Could you check a few things on this model? Use its own coordinates, in mm. Face numbers are marked on the shaded views. Coordinates: 2 decimals unless noted, no trailing zeros. Loops run counter-clockwise (first coordinate to the right, second up) from the corner with the lowest first, then second, coordinate; pieces in that order, holes last.
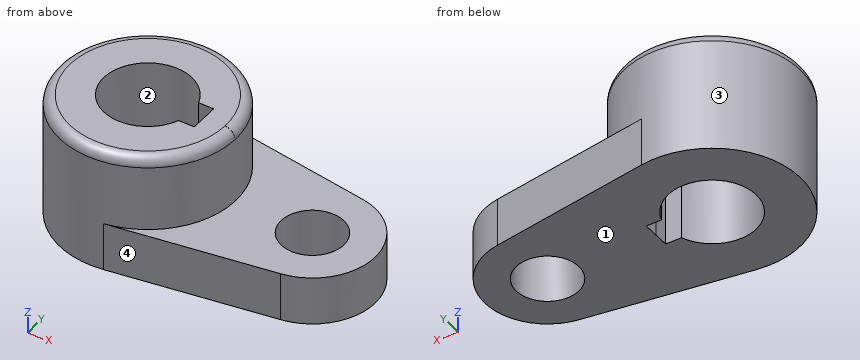
from build123d import *

# Parameters (mm, degrees)
F1_DEPTH = 15.7734
F2_DEPTH = 40.2336
F3_R     = 3.302


# Not quite as in the source:
# - a feature names something its author has since deleted; it is built from what else it names


with BuildPart() as f1:
    # F0 (on Top) → F1 (new body)
    with BuildSketch(Plane.XY):
        with BuildLine():
            ThreePointArc((28.5749057346, -0.0733979643), (28.5749764336, -0.0366990124), (28.575, 0))
            ThreePointArc((28.575, 0), (21.7196871584, 18.5684090525), (4.4430094671, 28.2274740612))
            ThreePointArc((4.4430094671, 28.2274740612), (-28.5749057039, 0.0734099128), (4.2979170796, -28.2499298013))
            ThreePointArc((4.2979170796, -28.2499298013), (21.6479758068, -18.6519641987), (28.5749057346, -0.0733979643))
        make_face()
        with BuildLine():
            Line((18.4686649637, 4.6872641706), (18.4984100104, -0.0475153147))
            Line((18.4984100104, -0.0475153147), (18.5293, -4.9645453691))
            Line((18.5293, -4.9645453691), (13.3852167998, -4.9968617623))
            ThreePointArc((13.3852167998, -4.9968617623), (-14.2863531341, 0.1810259026), (13.5075318215, 4.6560971147))
            Line((13.5075318215, 4.6560971147), (18.4686649637, 4.6872641706))
        make_face(mode=Mode.SUBTRACT)
        with BuildLine():
            ThreePointArc((4.4430094671, 28.2274740612), (21.7196871584, 18.5684090525), (28.575, 0))
            ThreePointArc((28.575, 0), (28.5749764336, -0.0366990124), (28.5749057346, -0.0733979643))
            ThreePointArc((28.5749057346, -0.0733979643), (21.6479758068, -18.6519641987), (4.2979170796, -28.2499298013))
            Line((4.2979170796, -28.2499298013), (56.9175468923, -20.2444300608))
            ThreePointArc((56.9175468923, -20.2444300608), (74.2947643422, -0.1870234197), (57.0132588055, 19.9529074106))
            Line((57.0132588055, 19.9529074106), (4.4430094671, 28.2274740612))
        make_face()
        with BuildLine():
            ThreePointArc((64.1348219431, -0.1386405993), (53.9617734053, -10.2986322201), (43.8148554597, -0.1125435453))
            ThreePointArc((43.8148554597, -0.1125435453), (53.9878704808, 10.0213510216), (64.1348219431, -0.1386405993))
        make_face(mode=Mode.SUBTRACT)
    extrude(amount=F1_DEPTH)

    # F0 (on Top) → F2 (join)
    with BuildSketch(Plane.XY):
        with BuildLine():
            ThreePointArc((28.5749057346, -0.0733979643), (28.5749764336, -0.0366990124), (28.575, 0))
            ThreePointArc((28.575, 0), (21.7196871584, 18.5684090525), (4.4430094671, 28.2274740612))
            ThreePointArc((4.4430094671, 28.2274740612), (-28.5749057039, 0.0734099128), (4.2979170796, -28.2499298013))
            ThreePointArc((4.2979170796, -28.2499298013), (21.6479758068, -18.6519641987), (28.5749057346, -0.0733979643))
        make_face()
        with BuildLine():
            Line((18.4686649637, 4.6872641706), (18.4984100104, -0.0475153147))
            Line((18.4984100104, -0.0475153147), (18.5293, -4.9645453691))
            Line((18.5293, -4.9645453691), (13.3852167998, -4.9968617623))
            ThreePointArc((13.3852167998, -4.9968617623), (-14.2863531341, 0.1810259026), (13.5075318215, 4.6560971147))
            Line((13.5075318215, 4.6560971147), (18.4686649637, 4.6872641706))
        make_face(mode=Mode.SUBTRACT)
    extrude(amount=F2_DEPTH)

    # F3
    f3_edges = [f1.edges().sort_by_distance(p)[0] for p in [
        (-4.297917, 28.24993, 40.2336),
    ]]
    fillet(f3_edges, radius=F3_R)


solid = f1.part
1) Imagine slicing it at D-D on x = 34. List the corners of the cut face in (y, z) for me, plus the area to 3 significant figures.
2) Imagine slicing it at B-B on z = 5.5. State how many separate pieces and enclosed holes the cut face has, plus the area to 3 significant figures.
3) If I drill on L1, parallel to X at y = 0, z = 13 (1 decimal); L2, parallel to Y at x = 0, z = 9 (1 decimal); L3, parallel to X at y = 8, z = 25, over which ranges is the centre line in solid material (lowest first)?
4) We'd pull the mould along Y, two halves only. Please class the marked faces 1, 2, 3 and 4: released by +Y, released by -Y, zero draft, split by the parting line, or undercut.
5) Will these pins go through, and if not, where does the flat tip stop? pin 1 (5 mm diameter, centred on y = 16, z = 24, fed in from -X); pin 2 (5 mm diameter, centred on y = 20.5, z = 14.5, fed in from -X); pin 3 (5 mm diameter, centred on x = 61.5, z = 12, fed in from +Y).
Solved:
1. outline: (-23.73, 0) - (23.58, 0) - (23.58, 15.77) - (-23.73, 15.77) - close
1. area: 746 mm2
2. separate pieces: 1
2. enclosed holes: 2
2. area: 3,590 mm2
3. L1: x = -28.6 to -14.3, 18.5 to 43.8, 64.1 to 74.3
3. L2: y = -28.6 to -14.3, 14.3 to 28.6
3. L3: x = -27.43 to -11.84, 11.84 to 27.43
4. face 1: zero draft
4. face 2: undercut
4. face 3: split by the parting line
4. face 4: released by -Y
5. pin 1: stops at x = -25.18
5. pin 2: stops at x = -22.19
5. pin 3: stops at y = 19.55
